```python
from build123d import *

# Parameters (mm, degrees)
F0_W      = 20
F0_H      = 20
F1_DEPTH  = 1770
F2_W      = 20
F2_H      = 20
F3_DEPTH  = 665
F4_W      = 20
F4_H      = 20
F5_DEPTH  = 520
F6_W      = 20
F6_H      = 20
F7_DEPTH  = 290
F8_W      = 20
F8_H      = 20
F9_DEPTH  = 645
F10_W     = 20
F10_H     = 20
F11_DEPTH = 645
F12_W     = 20
F12_H     = 20
F13_DEPTH = 920
F14_W     = 20
F14_H     = 20
F15_DEPTH = 1040
F16_W     = 20
F16_H     = 20
F17_DEPTH = 920
F18_W     = 20
F18_H     = 20
F19_DEPTH = 1030
F20_W     = 20
F20_H     = 20
F21_DEPTH = 920
F22_W     = 20
F22_H     = 20
F23_DEPTH = 645
F24_W     = 20
F24_H     = 20
F25_DEPTH = 790
F26_W     = 20
F26_H     = 20
F27_DEPTH = 500
F28_W     = 20
F28_H     = 20
F29_DEPTH = 645
F30_W     = 20
F30_H     = 20
F31_DEPTH = 270
F32_W     = 20
F32_H     = 20
F33_DEPTH = 645
F34_W     = 20
F34_H     = 20
F35_DEPTH = 680
F36_W     = 20
F36_H     = 20
F37_DEPTH = 645
F38_W     = 20
F38_H     = 20
F39_DEPTH = 270
F40_W     = 20
F40_H     = 20
F41_DEPTH = 1020
F43_W     = 20
F43_H     = 20
F44_DEPTH = 645
F42_W     = 20
F42_H     = 20
F45_DEPTH = 1020
F46_W     = 20
F46_H     = 20
F47_DEPTH = 790
F48_W     = 6
F48_H     = 80
F49_DEPTH = 1030
F50_W     = 6
F50_H     = 80
F51_DEPTH = 1030
F52_W     = 20
F52_H     = 20
F53_DEPTH = 480
F54_W     = 20
F54_H     = 20
F55_DEPTH = 1750
F56_W     = 20
F56_H     = 20
F57_DEPTH = 1030
F58_W     = 20
F58_H     = 20
F59_DEPTH = 500
F61_DEPTH = 6
F62_W     = 20
F62_H     = 20
F63_DEPTH = 1020
F64_W     = 20
F64_H     = 20
F65_DEPTH = 280
F66_W     = 20
F66_H     = 20
F67_DEPTH = 330


with BuildPart() as f1:
    # F0 (on Front) → F1 (new body)
    with BuildSketch(Plane.XZ):
        with Locations((10, 10)):
            Rectangle(F0_W, F0_H)
    extrude(amount=-F1_DEPTH)

    # F2 (on face) → F3 (join)
    with BuildSketch(Plane(origin=(0, 0, 0), x_dir=(0, -1, 0), z_dir=(-1, 0, 0))):
        with Locations((-10, 10)):
            Rectangle(F2_W, F2_H)
        with Locations((-1760, 10)):
            Rectangle(F2_W, F2_H)
    extrude(amount=F3_DEPTH)

    # F4 (on face) → F5 (join)
    with BuildSketch(Plane(origin=(0, 20, 0), x_dir=(-1, 0, 0), z_dir=(0, 1, 0))):
        with Locations((655, 10)):
            Rectangle(F4_W, F4_H)
    extrude(amount=F5_DEPTH)

    # F6 (on face) → F7 (join)
    with BuildSketch(Plane.XZ.offset(-1750)):
        with Locations((-655, 10)):
            Rectangle(F6_W, F6_H)
    extrude(amount=F7_DEPTH)

    # F8 (on face) → F9 (join, through all)
    with BuildSketch(Plane.YZ.offset(-645)):
        with Locations((530, 10)):
            Rectangle(F8_W, F8_H)
    extrude(amount=F9_DEPTH)

    # F10 (on face) → F11 (join, through all)
    with BuildSketch(Plane.YZ.offset(-645)):
        with Locations((1470, 10)):
            Rectangle(F10_W, F10_H)
    extrude(amount=F11_DEPTH)

    # F12 (on face) → F13 (join, through all)
    with BuildSketch(Plane.XZ.offset(-1460)):
        with Locations((-455, 10)):
            Rectangle(F12_W, F12_H)
    extrude(amount=F13_DEPTH)

    # F14 (on face) → F15 (join)
    with BuildSketch(Plane.XY.offset(20)):
        with Locations((10, 10)):
            Rectangle(F14_W, F14_H)
        with Locations((-655, 10)):
            Rectangle(F14_W, F14_H)
        with Locations((-655, 530)):
            Rectangle(F14_W, F14_H)
        with Locations((10, 1760)):
            Rectangle(F14_W, F14_H)
        with Locations((-655, 1470)):
            Rectangle(F14_W, F14_H)
        with Locations((-655, 1760)):
            Rectangle(F14_W, F14_H)
        with Locations((10, 1060)):
            Rectangle(F14_W, F14_H)
    extrude(amount=F15_DEPTH)

    # F16 (on face) → F17 (join, through all)
    with BuildSketch(Plane.XZ.offset(-1460)):
        with Locations((-655, 240)):
            Rectangle(F16_W, F16_H)
    extrude(amount=F17_DEPTH)

    # F18 (on face) → F19 (join, through all)
    with BuildSketch(Plane(origin=(0, 20, 0), x_dir=(-1, 0, 0), z_dir=(0, 1, 0))):
        with Locations((-10, 1050)):
            Rectangle(F18_W, F18_H)
    extrude(amount=F19_DEPTH)

    # F20 (on face) → F21 (join, through all)
    with BuildSketch(Plane(origin=(0, 540, 0), x_dir=(-1, 0, 0), z_dir=(0, 1, 0))):
        with Locations((655, 1050)):
            Rectangle(F20_W, F20_H)
    extrude(amount=F21_DEPTH)

    # F22 (on face) → F23 (join, through all)
    with BuildSketch(Plane(origin=(0, 0, 0), x_dir=(0, -1, 0), z_dir=(-1, 0, 0))):
        with Locations((-1060, 1050)):
            Rectangle(F22_W, F22_H)
    extrude(amount=F23_DEPTH)

    # F24 (on face) → F25 (join, through all)
    with BuildSketch(Plane(origin=(0, 0, 1040), x_dir=(1, 0, 0), z_dir=(0, 0, -1))):
        with Locations((-655, -1060)):
            Rectangle(F24_W, F24_H)
    extrude(amount=F25_DEPTH)

    # F26 (on face) → F27 (join, through all)
    with BuildSketch(Plane.XZ.offset(-520)):
        with Locations((-655, 1050)):
            Rectangle(F26_W, F26_H)
    extrude(amount=F27_DEPTH)

    # F28 (on face) → F29 (join, through all)
    with BuildSketch(Plane.YZ.offset(-645)):
        with Locations((10, 1050)):
            Rectangle(F28_W, F28_H)
    extrude(amount=F29_DEPTH)

    # F30 (on face) → F31 (join, through all)
    with BuildSketch(Plane(origin=(0, 1480, 0), x_dir=(-1, 0, 0), z_dir=(0, 1, 0))):
        with Locations((655, 240)):
            Rectangle(F30_W, F30_H)
    extrude(amount=F31_DEPTH)

    # F32 (on face) → F33 (join, through all)
    with BuildSketch(Plane.YZ.offset(-645)):
        with Locations((1760, 240)):
            Rectangle(F32_W, F32_H)
        with Locations((1060, 240)):
            Rectangle(F32_W, F32_H)
    extrude(amount=F33_DEPTH)

    # F34 (on face) → F35 (join, through all)
    with BuildSketch(Plane.XZ.offset(-1750)):
        with Locations((10, 240)):
            Rectangle(F34_W, F34_H)
    extrude(amount=F35_DEPTH)

    # F36 (on face) → F37 (join, through all)
    with BuildSketch(Plane.YZ.offset(-645)):
        with Locations((1760, 1050)):
            Rectangle(F36_W, F36_H)
    extrude(amount=F37_DEPTH)

    # F38 (on face) → F39 (join, through all)
    with BuildSketch(Plane(origin=(0, 1480, 0), x_dir=(-1, 0, 0), z_dir=(0, 1, 0))):
        with Locations((655, 1050)):
            Rectangle(F38_W, F38_H)
    extrude(amount=F39_DEPTH)

    # F40 (on face) → F41 (join, through all)
    with BuildSketch(Plane.XY.offset(20)):
        with Locations((-30, 10)):
            Rectangle(F40_W, F40_H)
    extrude(amount=F41_DEPTH)

    # F43 (on face) → F44 (join, through all)
    with BuildSketch(Plane.YZ.offset(-645)):
        with Locations((530, 1050)):
            Rectangle(F43_W, F43_H)
    extrude(amount=F44_DEPTH)

    # F42 (on face) → F45 (join, through all)
    with BuildSketch(Plane.XY.offset(20)):
        with Locations((-30, 530)):
            Rectangle(F42_W, F42_H)
    extrude(amount=F45_DEPTH)

    # F46 (on face) → F47 (join, through all)
    with BuildSketch(Plane.XY.offset(250)):
        with Locations((-30, 1060)):
            Rectangle(F46_W, F46_H)
    extrude(amount=F47_DEPTH)

    # F48 (on face) → F49 (join, through all)
    with BuildSketch(Plane.XZ.offset(-1050)):
        with Locations((-648, 640)):
            Rectangle(F48_W, F48_H)
    extrude(amount=F49_DEPTH)

    # F50 (on face) → F51 (join, through all)
    with BuildSketch(Plane.XZ.offset(-1050)):
        with Locations((-37, 640)):
            Rectangle(F50_W, F50_H)
    extrude(amount=F51_DEPTH)

    # F52 (on face) → F53 (join)
    with BuildSketch(Plane.XY.offset(1060)):
        with Locations((10, 10)):
            Rectangle(F52_W, F52_H)
        with Locations((10, 1060)):
            Rectangle(F52_W, F52_H)
        with Locations((10, 1760)):
            Rectangle(F52_W, F52_H)
        with Locations((-510, 10)):
            Rectangle(F52_W, F52_H)
        with Locations((-510, 1060)):
            Rectangle(F52_W, F52_H)
        with Locations((-510, 1760)):
            Rectangle(F52_W, F52_H)
    extrude(amount=F53_DEPTH)

    # F54 (on face) → F55 (join, through all)
    with BuildSketch(Plane.XZ.offset(-1750)):
        with Locations((-510, 1530)):
            Rectangle(F54_W, F54_H)
    extrude(amount=F55_DEPTH)

    # F56 (on face) → F57 (join, through all)
    with BuildSketch(Plane.XZ.offset(-1050)):
        with Locations((10, 1530)):
            Rectangle(F56_W, F56_H)
    extrude(amount=F57_DEPTH)

    # F58 (on face) → F59 (join, through all)
    with BuildSketch(Plane.YZ.offset(-500)):
        with Locations((10, 1530)):
            Rectangle(F58_W, F58_H)
        with Locations((1060, 1530)):
            Rectangle(F58_W, F58_H)
        with Locations((1760, 1530)):
            Rectangle(F58_W, F58_H)
    extrude(amount=F59_DEPTH)

    # F60 (on face) → F61 (join)
    with BuildSketch(Plane(origin=(0, 0, 0), x_dir=(1, 0, 0), z_dir=(0, 0, -1))):
        Polygon((-645, -100), (-565, -20), (-645, -20), align=None)
        Polygon((0, -100), (0, -20), (-80, -20), align=None)
        Polygon((-645, -440), (-645, -520), (-565, -520), align=None)
        Polygon((0, -520), (0, -440), (-80, -520), align=None)
        Polygon((0, -540), (-80, -540), (0, -620), align=None)
        Polygon((-445, -620), (-365, -540), (-445, -540), align=None)
        Polygon((-80, -1460), (0, -1460), (0, -1380), align=None)
        Polygon((-445, -1380), (-445, -1460), (-365, -1460), align=None)
        Polygon((0, -1560), (0, -1480), (-80, -1480), align=None)
        Polygon((-80, -1750), (0, -1750), (0, -1670), align=None)
        Polygon((-645, -1670), (-645, -1750), (-565, -1750), align=None)
        Polygon((-645, -1480), (-645, -1560), (-565, -1480), align=None)
    extrude(amount=-F61_DEPTH)

    # F62 (on face) → F63 (join, through all)
    with BuildSketch(Plane.XY.offset(20)):
        with Locations((10, 360)):
            Rectangle(F62_W, F62_H)
        with Locations((10, 760)):
            Rectangle(F62_W, F62_H)
    extrude(amount=F63_DEPTH)

    # F64 (on face) → F65 (join, through all)
    with BuildSketch(Plane(origin=(0, 770, 0), x_dir=(-1, 0, 0), z_dir=(0, 1, 0))):
        with Locations((-10, 430)):
            Rectangle(F64_W, F64_H)
    extrude(amount=F65_DEPTH)

    # F66 (on face) → F67 (join, through all)
    with BuildSketch(Plane(origin=(0, 20, 0), x_dir=(-1, 0, 0), z_dir=(0, 1, 0))):
        with Locations((-10, 430)):
            Rectangle(F66_W, F66_H)
    extrude(amount=F67_DEPTH)


solid = f1.part
```
Verification items for the finished model (mm, model axes). A direction names the side the tool comes from. Coordinates: 2 decimals unless noted, no trailing zeros. Loops run counter-clockwise (first coordinate to the right, second up) from the corner with the lowest first, then second, coordinate; pieces in that order, holes last. Notation, with made-up numbers: (56.5, -28) -> (99.5, -28) arc R29 ccw to (99.5, -4) -> close; hole circle Ø3 at (44, 81.5). An arc over 180 degrees is marked (long way). Answer in a Markdown table with one row per item.
1) Section check B-B (y = 1207.5). Record the cut outline in (x, z).
The answers:
| item | result |
|---|---|
| outline | (-665, 230) -> (-645, 230) -> (-645, 250) -> (-665, 250) -> close; (-665, 1040) -> (-645, 1040) -> (-645, 1060) -> (-665, 1060) -> close; (-520, 1520) -> (-500, 1520) -> (-500, 1540) -> (-520, 1540) -> close; (-465, 0) -> (-445, 0) -> (-445, 20) -> (-465, 20) -> close; (0, 0) -> (20, 0) -> (20, 20) -> (0, 20) -> close; (0, 230) -> (20, 230) -> (20, 250) -> (0, 250) -> close |
2) Section check A-A (z = 1101). Record the cut outline in (x, y).
The answers:
| item | result |
|---|---|
| outline | (-520, 0) -> (-500, 0) -> (-500, 20) -> (-520, 20) -> close; (-520, 1050) -> (-500, 1050) -> (-500, 1070) -> (-520, 1070) -> close; (-520, 1750) -> (-500, 1750) -> (-500, 1770) -> (-520, 1770) -> close; (0, 0) -> (20, 0) -> (20, 20) -> (0, 20) -> close; (0, 1050) -> (20, 1050) -> (20, 1070) -> (0, 1070) -> close; (0, 1750) -> (20, 1750) -> (20, 1770) -> (0, 1770) -> close |
3) Section check C-C (x = -598.5). Give the number of separate pieces and of enclosed holes in the cut face, and give its area (3 significant figures).
The answers:
| item | result |
|---|---|
| separate pieces | 10 |
| enclosed holes | 0 |
| area | 4,800 mm2 |
4) Depth check by flat-ended pin: P1, Ø22, axis at y = 527, z = 394, coming from the +X side; P2, Ø8, axis at y = 470, z = 1065.5, coming from the -X side. Enter the tip coordinate at first touch or a pass-through.
The answers:
| item | result |
|---|---|
| P1 | stops at x = -20 |
| P2 | passes through |
5) Access from +Z, -Z, +X, -X, +Y, -Y to the whole of each face (thin tool, end or side, straight path). Record for faces 4 (the face through (-623, 497, 6)), 5 (the face through (-39, 1419, 3)), 6 (the face through (-651, 799, 639)), 7 (the face through (-299, 1770, 1052)).
The answers:
| item | result |
|---|---|
| face 4 | +Z |
| face 5 | +Z, -Z |
| face 6 | -X |
| face 7 | +Z, -Z, +X, -X, +Y |
6) Scan lines: line 1 along Y through (x, z) = (-192.5, 1048); line 2 along X through (y, z) = (1217, 231.5); line 3 along Z through (x, y) = (-445.5, 595). Record each from-to range of solid material in increasing order. Write a range as from..to.
The answers:
| item | result |
|---|---|
| line 1 | y = 0..20, 520..540, 1050..1070, 1750..1770 |
| line 2 | x = -665..-645, 0..20 |
| line 3 | z = 0..20 |
7) Draft check along X on faces 1 (the face through (-23, 1727, 6)), 2 (the face through (-647, 1460, 63)), 3 (the face through (-665, 1471, 370)). Enter one of: released by +X, released by -X, zero draft, split by the parting line, or undercut.
The answers:
| item | result |
|---|---|
| face 1 | undercut |
| face 2 | zero draft |
| face 3 | released by -X |
